The model under review builds one solid part; all positions refer to its coordinate system, in mm. A direction names the side the tool comes from. Give positions to 0.01 mm unless a question says otherwise; leave off trailing zeros. Loops run counter-clockwise (first coordinate to the right, second up) from the corner with the lowest first, then second, coordinate; pieces in that order, holes last. Notation, with made-up numbers: M 62.25,-39 L 92.25,-39 A25 cw 92.25,-24 Z; hole C 68.5,4.25 d5. An arc over 180 degrees is marked long. Return JSON: item names as keys, results as strings. Group by question number.
```python
from build123d import *

# Parameters (mm, degrees)
Y_KSEKLIK_EKSTR_ZYON1_DEPTH      = 15
Y_KSEKLIK_EKSTR_ZYON1_DEPTH_BACK = 15
IZIM2_R                          = 7.5
KES_EKSTR_ZYON1_DEPTH            = 31
IZIM3_R                          = 7.5
IZIM3_R_2                        = 4
Y_KSEKLIK_EKSTR_ZYON2_DEPTH      = 11.5
Y_KSEKLIK_EKSTR_ZYON2_DEPTH_BACK = 11.5
IZIM4_R                          = 1.6
KES_EKSTR_ZYON2_DEPTH            = 18


with BuildPart() as part:
    # izim1 → Y_kseklik-Ekstr_zyon1 (new body, two sides)
    with BuildSketch(Plane.XY) as y_kseklik_ekstr_zyon1_sk:
        Polygon((-15.5, 6), (-8.5, 6), (-5, 11), (5, 11), (8.5, 6), (15.5, 6), (15.5, -4), (17, -5), (17, -11), (6, -11), (6, -10.5), (-6, -10.5), (-6, -11), (-17, -11), (-17, -5), (-15.5, -4), align=None)
    extrude(amount=Y_KSEKLIK_EKSTR_ZYON1_DEPTH)
    extrude(y_kseklik_ekstr_zyon1_sk.sketch, amount=-Y_KSEKLIK_EKSTR_ZYON1_DEPTH_BACK)

    # izim2 → Kes-Ekstr_zyon1 (cut, through all)
    with BuildSketch(Plane.XY.offset(15)):
        Circle(IZIM2_R)
    extrude(amount=-KES_EKSTR_ZYON1_DEPTH, mode=Mode.SUBTRACT)

    # izim3 → Y_kseklik-Ekstr_zyon2 (add, two sides)
    with BuildSketch(Plane.XY) as y_kseklik_ekstr_zyon2_sk:
        Circle(IZIM3_R)
        Circle(IZIM3_R_2, mode=Mode.SUBTRACT)
    extrude(amount=Y_KSEKLIK_EKSTR_ZYON2_DEPTH)
    extrude(y_kseklik_ekstr_zyon2_sk.sketch, amount=-Y_KSEKLIK_EKSTR_ZYON2_DEPTH_BACK)

    # izim4 → Kes-Ekstr_zyon2 (cut, through all)
    with BuildSketch(Plane(origin=(0, 6, 0), x_dir=(1, 0, 0), z_dir=(0, 1, 0))):
        with Locations((-12, 8.9)):
            Circle(IZIM4_R)
        with Locations((-12, -8.9)):
            Circle(IZIM4_R)
        with Locations((12, -8.9)):
            Circle(IZIM4_R)
        with Locations((12, 8.9)):
            Circle(IZIM4_R)
    extrude(amount=-KES_EKSTR_ZYON2_DEPTH, mode=Mode.SUBTRACT)


solid = part.part
```
(1) Mouldability with a two-part tool opening along Z and no side actions: class faces 4 (the flat face through (-4, -7, -15)), 5 (the flat face through (-11, -11, 0)), 6 (the cylindrical face through (-13.18, -2.38, 7.82)) as released by +Z, released by -Z, zero draft, split by the parting line, or undercut.
(2) For probe 1 along Z at (x, y) = (12, -3.5); probe 2 along X at (y, z) = (-6, 8.9); probe 3 along X at (y, z) = (2.5, 8), list the stretches that pass through material, from the lowest coordinate up.
(3) For pin 1 (1 mm diameter, centred on y = -0.5, z = 9, fed in from +X); pin 2 (12 mm diameter, centred on y = 7, z = -3, fed in from -X); pin 3 (2 mm diameter, centred on x = 11, z = -6.5, fed in from +Y), all flat-tipped, find the tip position at first contact; note any pin that passes through.
(4) Add section D-D (x = -12). Write out the cut boundary in (y, z).
(5) Add section C-C (y = 0). Write out the cut boundary in (x, z).
(6) Add section B-B (z = 8.9). Write out the cut boundary in (x, y), and give its area (3 significant figures).
(7) Add section A-A (x = 0). Write out the cut boundary in (y, z), and give its area (3 significant figures).
(8) For faces 1 (the flat face through (15.5, 1, 0)), 2 (the cylindrical face through (-7.493, 0.33, 13.274)), 3 (the flat face through (-12, 6, 0)), list the 3-axis set-ups (+Z, -Z, +X, -X, +Y, -Y) from which the entire face can be reached by the end or side of a thin tool; tool diameter is ignored.
Verdict:
{
 "1": {"face 4": "released by -Z", "face 5": "zero draft", "face 6": "undercut"},
 "2": {"probe 1": "z = -15 to -10.5, -7.3 to 7.3, 10.5 to 15", "probe 2": "x = -17 to -13.6, -10.4 to 10.4, 13.6 to 17", "probe 3": "x = -15.5 to -13.32, -10.68 to -3.12, 3.12 to 10.68, 13.32 to 15.5"},
 "3": {"pin 1": "stops at x = 15.5", "pin 2": "stops at x = -15.5", "pin 3": "stops at y = 6"},
 "4": {"outline": "M -11,-15 L 6,-15 L 6,-10.5 L -11,-10.5 Z; M -11,-7.3 L 6,-7.3 L 6,7.3 L -11,7.3 Z; M -11,10.5 L 6,10.5 L 6,15 L -11,15 Z"},
 "5": {"outline": "M -15.5,-15 L -7.5,-15 L -7.5,-11.5 L -4,-11.5 L -4,11.5 L -7.5,11.5 L -7.5,15 L -15.5,15 Z; M 4,-11.5 L 7.5,-11.5 L 7.5,-15 L 15.5,-15 L 15.5,15 L 7.5,15 L 7.5,11.5 L 4,11.5 Z; hole C -12,-8.9 d3.2; hole C -12,8.9 d3.2; hole C 12,-8.9 d3.2; hole C 12,8.9 d3.2"},
 "6": {"outline": "M -17,-11 L -13.6,-11 L -13.6,6 L -15.5,6 L -15.5,-4 L -17,-5 Z; M -10.4,-11 L -6,-11 L -6,-10.5 L 6,-10.5 L 6,-11 L 10.4,-11 L 10.4,6 L 8.5,6 L 5,11 L -5,11 L -8.5,6 L -10.4,6 Z; M 13.6,-11 L 17,-11 L 17,-5 L 15.5,-4 L 15.5,6 L 13.6,6 Z; hole C 0,0 d8", "area": "449 mm²"},
 "7": {"outline": "M -10.5,-15 L -7.5,-15 L -7.5,-11.5 L -4,-11.5 L -4,11.5 L -7.5,11.5 L -7.5,15 L -10.5,15 Z; M 4,-11.5 L 7.5,-11.5 L 7.5,-15 L 11,-15 L 11,15 L 7.5,15 L 7.5,11.5 L 4,11.5 Z", "area": "356 mm²"},
 "8": {"face 1": "+Z, -Z, +X, +Y", "face 2": "+Z", "face 3": "+Z, -Z, -X, +Y"}
}
